```python
from build123d import *

# Parameters (mm, degrees)
EXTRUDE_THIN1_DEPTH = 100
SKETCH2_R           = 2
CUT_EXTRUDE1_DEPTH  = 36.197996578
CHAMFER1_SIZE       = 20
SKETCH3_R           = 3.25
CUT_EXTRUDE2_DEPTH  = 4.125


with BuildPart() as part:
    # Sketch1 → Extrude-Thin1 (new body)
    with BuildSketch(Plane(origin=(0, 0, 0), x_dir=(0, 0, -1), z_dir=(1, 0, 0))):
        Polygon((0, 0), (32.072996578, 0), (32.072996578, 38.1), (35.197996578, 38.1), (35.197996578, -3.125), (0, -3.125), align=None)
    extrude(amount=EXTRUDE_THIN1_DEPTH)

    # Sketch2 → Cut-Extrude1 (cut, through all)
    with BuildSketch(Plane(origin=(0, 0, -35.197996578), x_dir=(-1, 0, 0), z_dir=(0, 0, -1))):
        with Locations(Location((-40, 20, 0), (0, 0, 180))):  # turned: the seam where the file's is
            Circle(SKETCH2_R)
        with Locations((-60, 20)):
            Circle(SKETCH2_R)
    extrude(amount=-CUT_EXTRUDE1_DEPTH, mode=Mode.SUBTRACT)

    # Chamfer1
    chamfer1_edges = [part.edges().sort_by_distance(p)[0] for p in [
        (0, 38.1, -33.635496578),
        (100, 38.1, -33.635496578),
    ]]
    chamfer(chamfer1_edges, length=CHAMFER1_SIZE)

    # Sketch3 → Cut-Extrude2 (cut, through all)
    with BuildSketch(Plane(origin=(0, 0, 0), x_dir=(-1, 0, 0), z_dir=(0, 1, 0))):
        with Locations(Location((-80, -16.036498289, 0), (0, 0, 90))):  # turned: the seam where the file's is
            Circle(SKETCH3_R)
        with Locations(Location((-20, -16.036498289, 0), (0, 0, 270))):  # turned: the seam where the file's is
            Circle(SKETCH3_R)
    extrude(amount=-CUT_EXTRUDE2_DEPTH, mode=Mode.SUBTRACT)


solid = part.part
```
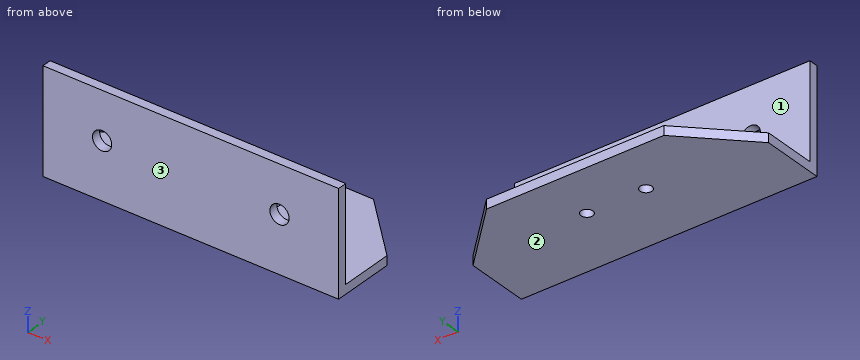
The listing builds one solid part. Answer for the finished solid, in the listing's coordinates (mm). Face numbers are marked on the shaded views. Coordinates: 2 decimals unless noted, no trailing zeros. Order: outer loops, then holes, each group sorted by start corner. A loop starts at its lowest first (then second) coordinate and runs counter-clockwise, first axis right, second up. Notation, with made-up numbers: M 9,30 L 44,30 A18 cw 44,36 Z; hole C 46,50 d2. An arc over 180 degrees is marked long. Answer as a JSON object with one key per item and string values. Group by question number.
1. Section D-D on x = 29 is taken. Write down the section's boundary in (y, z) (3 decimals), then the cut area to 3 significant figures.
2. Straight lines are drawn through the part: line 1 (Z direction, x = 20, y = -1); line 2 (Y direction, x = 40, z = -33.7) (3 decimals); line 3 (Z direction, x = 30, y = 8). For each, find the intervals that lie inside material, in ascending order.
3. Section C-C on z = -17.5 is taken. Write down the section's boundary in (x, y) (3 decimals), then the cut area to 3 significant figures.
4. Section A-A on x = 40 is taken. Write down the section's boundary in (y, z) (3 decimals), then the cut area to 3 significant figures.
5. Determine the mould class of the marked faces 1, 2 and 3 for opening direction Y: released by +Y, released by -Y, zero draft, split by the parting line, or undercut.
6. Section B-B on y = 20 is taken. Write down the section's boundary in (x, z).
7. Flat-ended cylindrical pins translate along their axes: P1, Ø2, axis at x = 16.5, z = -21.5, coming from the +Y side; P2, Ø6, axis at x = 20, z = -16.04, coming from the -Y side; P3, Ø4.5, axis at x = 40, y = 20, coming from the +Z side; P4, Ø6.5, axis at x = 60, y = 20, coming from the -Z side. Find the tip coordinate at first contact, or state that the pin passes through.
Values follow:
{
 "1": {"outline": "M -3.125,-35.198 L 38.1,-35.198 L 38.1,-32.073 L 0,-32.073 L 0,0 L -3.125,0 Z", "area": "229 mm2"},
 "2": {"line 1": "-35.2 to -19.29, -12.79 to 0", "line 2": "-3.125 to 18, 22 to 38.1", "line 3": "-35.2 to -32.07"},
 "3": {"outline": "M 0,-3.125 L 17.098,-3.125 L 17.098,0 L 0,0 Z; M 22.902,-3.125 L 77.098,-3.125 L 77.098,0 L 22.902,0 Z; M 82.902,-3.125 L 100,-3.125 L 100,0 L 82.902,0 Z", "area": "276 mm2"},
 "4": {"outline": "M -3.125,-35.198 L 18,-35.198 L 18,-32.073 L 0,-32.073 L 0,0 L -3.125,0 Z; M 22,-35.198 L 38.1,-35.198 L 38.1,-32.073 L 22,-32.073 Z", "area": "217 mm2"},
 "5": {"face 1": "released by +Y", "face 2": "zero draft", "face 3": "released by -Y"},
 "6": {"outline": "M 1.9,-35.2 L 38,-35.2 L 38,-32.07 L 1.9,-32.07 Z; M 42,-35.2 L 58,-35.2 L 58,-32.07 L 42,-32.07 Z; M 62,-35.2 L 98.1,-35.2 L 98.1,-32.07 L 62,-32.07 Z"},
 "7": {"P1": "y = 0", "P2": "through", "P3": "z = -32.07", "P4": "z = -35.2"}
}
